Read the model definition and answer for the solid it produces. Units are mm, in the model's axes. A direction names the side the tool comes from. Give positions to 0.01 mm unless a question says otherwise; leave off trailing zeros. Order: outer loops, then holes, each group sorted by start corner. A loop starts at its lowest first (then second) coordinate and runs counter-clockwise, first axis right, second up.
```python
from build123d import *

# Parameters (mm, degrees)
SKETCH_W        = 30
SKETCH_H        = 30
SKETCH_R        = 8
SKETCH_R_2      = 1.6
PAD_DEPTH       = 6
SKETCH002_R     = 3
POCKET_DEPTH    = 15.001
COPYSKETCH003_W = 7
COPYSKETCH003_H = 5
PAD001_DEPTH    = 6
COPYSKETCH004_R = 1.55
POCKET001_DEPTH = 5
FILLET_R        = 4


with BuildPart() as part:
    # Sketch → Pad (new body)
    with BuildSketch(Plane.XY):
        Rectangle(SKETCH_W, SKETCH_H)
        Circle(SKETCH_R, mode=Mode.SUBTRACT)
        with Locations((-11, 11)):
            Circle(SKETCH_R_2, mode=Mode.SUBTRACT)
        with Locations((11, 11)):
            Circle(SKETCH_R_2, mode=Mode.SUBTRACT)
        with Locations((-11, -11)):
            Circle(SKETCH_R_2, mode=Mode.SUBTRACT)
        with Locations((11, -11)):
            Circle(SKETCH_R_2, mode=Mode.SUBTRACT)
    extrude(amount=PAD_DEPTH)

    # Sketch001 → Revolution (revolve)
    with BuildSketch(Plane.XZ):
        Polygon((9.2, 6), (9.2, 16.321539), (8, 18.4), (8, 20.9), (8.5, 21.4), (8, 21.9), (8, 22.9), (8.5, 23.4), (8, 23.9), (8, 24.9), (8.5, 25.4), (8, 25.9), (8, 27.4), (6.8, 27.4), (6.8, 18.078461), (8, 16), (8, 6), align=None)
    revolve(axis=Axis((0, 0, 0), (0, 0, 1)))

    # Sketch002 → Pocket (cut, through all)
    with BuildSketch(Plane.XZ):
        with Locations((0, 11)):
            Circle(SKETCH002_R)
    extrude(amount=POCKET_DEPTH, mode=Mode.SUBTRACT)

    # CopySketch003 → Pad001 (join)
    with BuildSketch(Plane(origin=(0, 0, 0), x_dir=(1, 0, 0), z_dir=(0, 0, -1))):
        with Locations((-17.5, -12.5)):
            Rectangle(COPYSKETCH003_W, COPYSKETCH003_H)
        with Locations((17.5, -12.5)):
            Rectangle(COPYSKETCH003_W, COPYSKETCH003_H)
    extrude(amount=-PAD001_DEPTH)

    # CopySketch004 → Pocket001 (cut)
    with BuildSketch(Plane.XZ.offset(-10)):
        with Locations((-18, 3)):
            Circle(COPYSKETCH004_R)
        with Locations((18, 3)):
            Circle(COPYSKETCH004_R)
    extrude(amount=-POCKET001_DEPTH, mode=Mode.SUBTRACT)

    # Fillet
    fillet_edges = [part.edges().sort_by_distance(p)[0] for p in [
        (-15, -15, 3),
        (15, -15, 3),
    ]]
    fillet(fillet_edges, radius=FILLET_R)


solid = part.part
```
1) Consider L1, parallel to Y at x = -11, z = 2; L2, parallel to Z at x = 18, y = 11.6; L3, parallel to Y at x = 0, z = 3.75. Determine where each line is inside the solid, lowest interval first.
Final values:
L1: y = -15 to -12.6, -9.4 to 9.4, 12.6 to 15
L2: z = 0 to 1.45, 4.55 to 6
L3: y = -15 to -8, 8 to 15
2) The part is cut by section D-D on x = 13.5. Determine the outline of the cut face in (y, z).
Final values:
outline: (-14.12, 0) - (15, 0) - (15, 6) - (-14.12, 6) - close
3) For a pull along Z with two mould halves and no side action, classify faces 1 (the face through (-13.859, -13.797, 3.042)), 2 (the face through (-1.73, -7.81, 19.67)) as released by +Z, released by -Z, zero draft, split by the parting line, or undercut.
Final values:
face 1: zero draft
face 2: undercut
4) The part is cut by section C-C on z = 7. Determine the outline of the cut face in (x, y).
Final values:
outline: circle Ø18.4 at (0, 0); hole circle Ø16 at (0, 0)
5) Given pin 1 (14.5 mm diameter, centred on x = 0, y = 0, fed in from -Z); pin 2 (6 mm diameter, centred on x = -7, z = 11.5, fed in from +Y); pin 3 (7 mm diameter, centred on x = 0, z = 11, fed in from +Y), each flat-ended and moving along its own axis, determine where each tip first touches the part or whether it passes through.
Final values:
pin 1: stops at z = 17.3
pin 2: stops at y = 8.28
pin 3: stops at y = 9.2
6) The part is cut by section A-A on y = 11. Determine the outline of the cut face in (x, z).
Final values:
outline: (-21, 0) - (-12.6, 0) - (-12.6, 6) - (-21, 6) - close; (-9.4, 0) - (9.4, 0) - (9.4, 6) - (-9.4, 6) - close; (12.6, 0) - (21, 0) - (21, 6) - (12.6, 6) - close; hole circle Ø3.1 at (-18, 3); hole circle Ø3.1 at (18, 3)
7) A tool of negligible diameter and unlimited length cuts with its end or side. For faces 3 (the face through (4.946, 7.757, 11.233)), 4 (the face through (-1.73, -7.81, 22.41)), 5 (the face through (4.301, 6.746, 7.888)), 6 (the face through (-16.568, 12.465, 2.406)), 7 (the face through (15, -1, 3)), from which of +Z, -Z, +X, -X, +Y, -Y can it reach the whole face along a straight path? Write none if from no direction.
Final values:
face 3: +Z
face 4: none
face 5: -Z
face 6: +Y, -Y
face 7: +Z, -Z, +X, -Y
8) The part is cut by section B-B on z = 3. Determine the outline of the cut face in (x, y).
Final values:
outline: (-21, 10) - (-19.55, 10) - (-19.55, 15) - (-21, 15) - close; (-16.45, 10) - (-15, 10) - (-15, -11) arc R4 ccw to (-11, -15) - (11, -15) arc R4 ccw to (15, -11) - (15, 10) - (16.45, 10) - (16.45, 15) - (-16.45, 15) - close; (19.55, 10) - (21, 10) - (21, 15) - (19.55, 15) - close; hole circle Ø3.2 at (-11, -11); hole circle Ø3.2 at (-11, 11); hole circle Ø16 at (0, 0); hole circle Ø3.2 at (11, -11); hole circle Ø3.2 at (11, 11)
